Here's the drawing with two shaded views (mm, measured from the low corner). I have some questions. Round coordinates to 2 decimals unless told otherwise and drop trailing zeros. Order: outer loops, then holes, each group sorted by start corner. A loop starts at its lowest first (then second) coordinate and runs counter-clockwise, first axis right, second up. Notation, with made-up numbers: (50.5, 19.5) - (77.5, 19.5) arc R19 ccw to (77.5, 56.5) - close; hole circle Ø5 at (26, -35.75). An arc over 180 degrees is marked (long way). One line per item, written item: value.
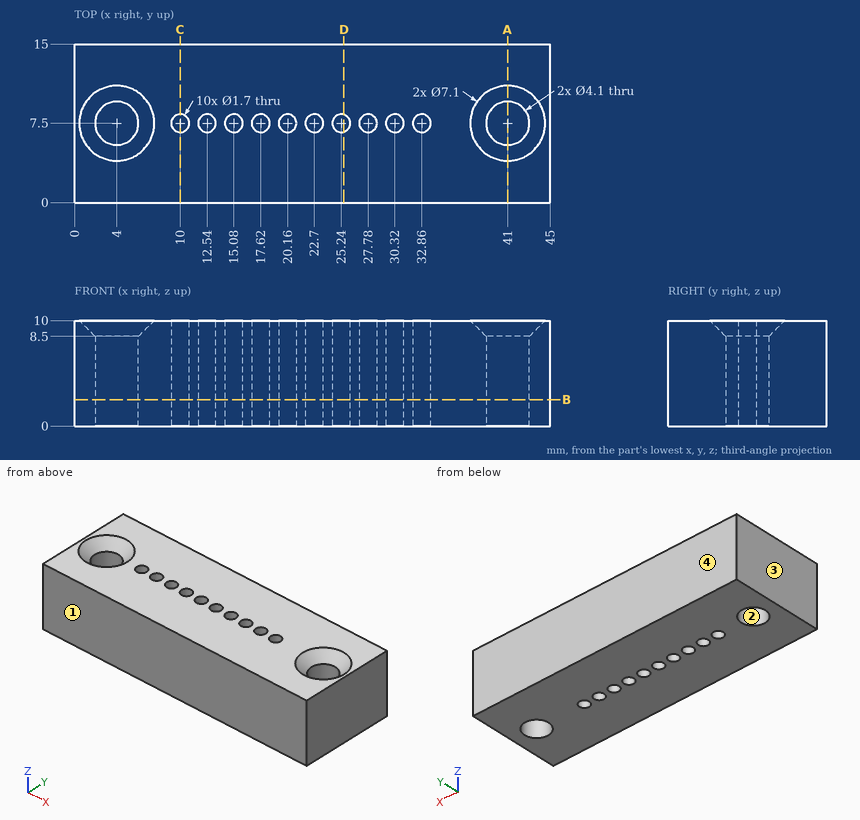
Q1. Will these pins go through, and if not, where does the flat tip stop? pin 1 (1.5 mm diameter, centred on x = 32.86, y = 7.5, fed in from -Z); pin 2 (2.5 mm diameter, centred on x = 17.62, y = 7.5, fed in from +Z).
Results list:
pin 1: through
pin 2: z = 10
Q2. If we section it at D-D, the plane x = 25.5: Please give me the cut outline in (y, z), then the cut area to 3 significant figures.
Results list:
outline: (0, 0) - (6.69, 0) - (6.69, 10) - (0, 10) - close; (8.31, 0) - (15, 0) - (15, 10) - (8.31, 10) - close
area: 134 mm²
Q3. If we section it at B-B, the plane z = 2.5: Give the number of separate pieces and of enclosed holes in the cut face, then the cut area to 3 significant figures.
Results list:
separate pieces: 1
enclosed holes: 12
area: 626 mm²
Q4. If we section it at A-A, the plane x = 41: Please give me the cut outline in (y, z).
Results list:
outline: (0, 0) - (5.45, 0) - (5.45, 8.5) - (3.95, 10) - (0, 10) - close; (9.55, 0) - (15, 0) - (15, 10) - (11.05, 10) - (9.55, 8.5) - close
Q5. If we section it at C-C, the plane x = 10: Please give me the cut outline in (y, z).
Results list:
outline: (0, 0) - (6.65, 0) - (6.65, 10) - (0, 10) - close; (8.35, 0) - (15, 0) - (15, 10) - (8.35, 10) - close
Q6. We'd pull the mould along Y, two halves only. Please class the marked faces 1, 2, 3 and 4: released by +Y, released by -Y, zero draft, split by the parting line, or undercut.
Results list:
face 1: released by -Y
face 2: undercut
face 3: zero draft
face 4: released by +Y
Q7. If I drill on line 1 along Y through (x, z) = (15.08, 7); line 2 along Y through (x, z) = (41, 5.5); line 3 along X through (y, z) = (9, 4.5), over which ranges is the centre line in solid material (lowest first)?
Results list:
line 1: 0 to 6.65, 8.35 to 15
line 2: 0 to 5.45, 9.55 to 15
line 3: 0 to 2.6, 5.4 to 39.6, 42.4 to 45
